Autodesk Inventor part; units mm, degrees
ref_plane "YZ Plane" through (0, 0, 0) normal (1, 0, 0) x (0, 1, 0)
ref_plane "XZ Plane" through (0, 0, 0) normal (0, 1, 0) x (-1, 0, 0)
ref_plane "XY Plane" through (0, 0, 0) normal (0, 0, 1) x (1, 0, 0)
sketch "Sketch1" plane through (0, 0, 0) normal (0, 0, 1) x (1, 0, 0)
  line L0 (0, 0) -> (90, 0)
  line L1 (90, 0) -> (90, -120)
  line L2 (90, -120) -> (0, -120)
  line L3 (0, -120) -> (0, 0)
  dimension "d0" = 90
  dimension "d1" = 120
extrude "Extrusion1" add sketch "Sketch1" along normal blind 3.175
sketch "Sketch2" plane through (0, 0, 3.175) normal (0, 0, 1) x (1, 0, 0)
  point P0 (0, 0)
sketch "Sketch3" plane through (0, 0, 3.175) normal (0, 0, 1) x (1, 0, 0)
  line L0 (0, -120) -> (90, -120)
  line L1 (0, 0) -> (90, 0)
  line L2 (90, 0) -> (90, -120)
  line L3 (90, -120) -> (0, -120)
  line L4 (0, -120) -> (0, 0)
  line L5 (90, 0) -> (0, 0)
  line L6 (0, 0) -> (3.175, 0)
  line L7 (90, -120) -> (90, -116.825)
  line L8 (90, -120) -> (90, 0)
  line L9 (3.175, -3.175) -> (86.825, -3.175)
  line L10 (86.825, -3.175) -> (86.825, -116.825)
  line L11 (86.825, -116.825) -> (3.175, -116.825)
  line L12 (3.175, -116.825) -> (3.175, -3.175)
  dimension "d4" = 3.175
  dimension "d5" = 3.175
  dimension "d7" = 3.175
extrude "Extrusion2" add sketch "Sketch3" along normal blind 30
sketch "Sketch4" plane through (0, 0, 33.175) normal (0, 0, 1) x (1, 0, 0)
  line L0 (0, 0) -> (90, 0)
  line L1 (0, -120) -> (0, 0)
  line L2 (0, 0) -> (0, -120)
  line L3 (90, -120) -> (0, -120)
  line L4 (0, -120) -> (90, -120)
  line L5 (90, -120) -> (90, 0)
  line L6 (90, 0) -> (88, 0)
  line L7 (88, 0) -> (88, -116.825)
  line L8 (3.175, -116.825) -> (86.825, -116.825)
  line L9 (88, -116.825) -> (3.175, -116.825)
  line L10 (3.175, -116.825) -> (2, -116.825)
  line L11 (2, -116.825) -> (2, 0)
  line L12 (2, 0) -> (0, 0)
  dimension "d10" = 2
  dimension "d11" = 1.175
extrude "Extrusion3" add sketch "Sketch4" along normal blind 2.75 contours L0 L11 L10 L8 L9 L7 L5 L3 L1
sketch "Sketch5" plane through (0, 0, 35.925) normal (0, 0, 1) x (1, 0, 0)
  line L0 (0, 0) -> (90, 0)
  line L1 (0, 0) -> (3.175, 0)
  line L2 (86.825, -3.175) -> (3.175, -3.175)
  line L3 (3.175, -116.825) -> (86.825, -116.825)
  line L4 (3.175, 0) -> (3.175, -116.825)
  line L5 (3.175, -116.825) -> (86.825, -116.825)
  line L6 (86.825, -116.825) -> (86.825, 0)
  line L7 (90, 0) -> (90, -120)
  line L8 (86.825, 0) -> (90, 0)
  line L9 (90, 0) -> (90, -120)
  line L10 (90, -120) -> (0, -120)
  line L11 (90, -120) -> (0, -120)
  line L12 (0, -120) -> (0, 0)
  line L13 (0, -120) -> (0, 0)
  line L14 (0, 0) -> (3.175, 0)
extrude "Extrusion4" add sketch "Sketch5" along normal blind 2 contours L0 L4 L3 L6 L7 L10 L12
sketch "Sketch6" plane through (0, 0, 0) normal (0, 1, 0) x (1, 0, 0)
  line L0 (3.175, -3.175) -> (86.825, -3.175)
  line L1 (3.175, -3.175) -> (3.175, -33.175)
  line L2 (86.825, -3.175) -> (3.175, -3.175)
  line L3 (3.175, -3.175) -> (45, -3.175)
  line L4 (45, -13.925) -> (6.3314, -13.925)
  line L5 (6.3314, -13.925) -> (34.8314, -13.925)
  line L6 (34.8314, -13.925) -> (34.8314, -3.175)
  line L7 (34.8314, -3.175) -> (6.3314, -3.175)
  line L8 (6.3314, -3.175) -> (6.3314, -13.925)
  point P0 (0, 0)
  dimension "d16" = 10.75
  dimension "d18" = 28.5
  dimension "d46" = 3.1564
extrude "Extrusion5" cut sketch "Sketch6" against normal blind 3.175
sketch "Sketch7" plane through (0, 0, 3.175) normal (0, 0, 1) x (1, 0, 0)
  line L0 (0, -120) -> (90, -120)
  line L1 (90, -120) -> (34.437, -120)
  line L2 (34.437, -120) -> (34.437, -75.55)
  line L3 (34.437, -75.55) -> (90, -75.55)
  line L4 (90, -75.55) -> (90, -120)
  line L5 (90, -120) -> (34.437, -120)
  line L6 (62.2185, -120) -> (62.2185, -97.575)
  dimension "d22" = 55.563
  dimension "d23" = 44.45
  dimension "d24" = 22.425
hole "Hole1" at (62.2185, -97.575, 3.175) direction (0, 0, -1) diameter 10 end through all
sketch "Sketch8" plane through (0, 0, 3.175) normal (0, 0, 1) x (1, 0, 0)
  circle A0 centre (62.2185, -97.575) radius 5
  line L0 (62.2185, -97.575) -> (71.7185, -97.575)
  line L1 (71.7185, -97.575) -> (71.7185, -88.075)
  line L2 (71.7185, -88.075) -> (52.7185, -88.075)
  line L3 (52.7185, -88.075) -> (52.7185, -107.075)
  line L4 (52.7185, -107.075) -> (71.7185, -107.075)
  line L5 (71.7185, -107.075) -> (71.7185, -88.075)
  point P0 (0, 0)
  dimension "d32" = 9.5
  dimension "d33" = 9.5
  dimension "d34" = 19
  dimension "d35" = 19
hole "Hole2" at (52.7185, -88.075, 3.175) at (71.7185, -88.075, 3.175) at (71.7185, -107.075, 3.175) at (52.7185, -107.075, 3.175) direction (0, 0, -1) diameter 3 end through all
fillet "Fillet1" radius 2 2 edges at (0, 0, 18.9625) (90, 0, 18.9625)
fillet "Fillet2" radius 2 2 edges at (0, -120, 18.9625) (90, -120, 18.9625)
fillet "Fillet3" radius 2 1 edges at (45, 0, 33.175)
properties part number "BatteryBox"
Work out the finished part from the listing and answer in its coordinate system (mm). A direction names the side the tool comes from. Give positions to 0.01 mm unless a question says otherwise; leave off trailing zeros. Loops run counter-clockwise (first coordinate to the right, second up) from the corner with the lowest first, then second, coordinate; pieces in that order, holes last. Notation, with made-up numbers: (47, 81.25) -> (86, 81.25) arc R19 cw to (86, 88.25) -> close; hole circle Ø1 at (18.25, -22). An arc over 180 degrees is marked (long way). Use a Markdown table: item, result. Add a question column.
1) Consider line 1 along X through (y, z) = (-57, 10.5) (3 decimals); line 2 along X through (y, z) = (-43, 33.5); line 3 along Y through (x, z) = (84.5, 27.5) (3 decimals). Determine where each line is inside the solid, lowest interval first.
2) The part is cut by section D-D, the plane y = -29. Determine the outline of the cut face in (x, z) (3 decimals), plus the area to 3 significant figures.
3) The part is cut by section C-C, the plane y = -107. Determine the outline of the cut face in (x, z) (3 decimals), plus the area to 3 significant figures.
4) The part is cut by section A-A, the plane x = 20. Determine the outline of the cut face in (y, z) (3 decimals), plus the area to 3 significant figures.
5) This flat-tipped pin is pushed along its axis until it touches: P1, Ø5, axis at x = 71.72, y = -107.08, coming from the +Z side (3 decimals). Where does it stop, or does it pass through?
6) Which of the six approach directions +Z, -Z, +X, -X, +Y, -Y give full straight-line access (tool end or side, diameter ignored) to faces 3 (the cylindrical face through (53.631, -105.885, 1.565)), 4 (the flat face through (86.825, -59, 18)), 5 (the flat face through (21, -2, 13.925))?
7) The part is cut by section B-B, the plane z = 16.5. Determine the outline of the cut face in (x, y) (1 decimal).
8) For a pull along X with two mould halves and no side action, classify faces 1 (the flat face through (6.331, -2, 8)), 2 (the flat face through (44, -59, 0)) as +X half, -X half, draft (parallel to the pull), parting line (faces both ways), or undercut.
Reported:
| question | item | result |
|---|---|---|
| 1 | line 1 | x = 0 to 3.175, 86.825 to 90 |
| 1 | line 2 | x = 0 to 2, 88 to 90 |
| 1 | line 3 | y = -120 to -116.825, -3.175 to 0 |
| 2 | outline | (0, 0) -> (90, 0) -> (90, 37.925) -> (86.825, 37.925) -> (86.825, 35.925) -> (88, 35.925) -> (88, 33.175) -> (86.825, 33.175) -> (86.825, 3.175) -> (3.175, 3.175) -> (3.175, 33.175) -> (2, 33.175) -> (2, 35.925) -> (3.175, 35.925) -> (3.175, 37.925) -> (0, 37.925) -> close |
| 2 | area | 500 mm^2 |
| 3 | outline | (0, 0) -> (51.22, 0) -> (51.22, 3.175) -> (3.175, 3.175) -> (3.175, 33.175) -> (2, 33.175) -> (2, 35.925) -> (3.175, 35.925) -> (3.175, 37.925) -> (0, 37.925) -> close; (54.217, 0) -> (70.22, 0) -> (70.22, 3.175) -> (54.217, 3.175) -> close; (73.217, 0) -> (90, 0) -> (90, 37.925) -> (86.825, 37.925) -> (86.825, 35.925) -> (88, 35.925) -> (88, 33.175) -> (86.825, 33.175) -> (86.825, 3.175) -> (73.217, 3.175) -> close |
| 3 | area | 481 mm^2 |
| 4 | outline | (-120, 0) -> (0, 0) -> (0, 3.175) -> (-116.825, 3.175) -> (-116.825, 37.925) -> (-120, 37.925) -> close; (-3.175, 13.925) -> (0, 13.925) -> (0, 31.175) arc R2 ccw to (-2, 33.175) -> (-3.175, 33.175) -> close |
| 4 | area | 552 mm^2 |
| 5 | P1 | stops at z = 3.175 |
| 6 | face 3 | +Z, -Z |
| 6 | face 4 | +Z |
| 6 | face 5 | +Y |
| 7 | outline | (0, -118) arc R2 ccw to (2, -120) -> (88, -120) arc R2 ccw to (90, -118) -> (90, -2) arc R2 ccw to (88, 0) -> (2, 0) arc R2 ccw to (0, -2) -> close; hole (3.2, -116.8) -> (86.8, -116.8) -> (86.8, -3.2) -> (3.2, -3.2) -> close |
| 8 | face 1 | undercut |
| 8 | face 2 | draft |
